CAD build for the part. Positions are in the model's coordinates, mm. A direction names the side the tool comes from. Give positions to 0.01 mm unless a question says otherwise; leave off trailing zeros. Order: outer loops, then holes, each group sorted by start corner. A loop starts at its lowest first (then second) coordinate and runs counter-clockwise, first axis right, second up. Notation, with made-up numbers: (-14, 30.5) -> (23, 30.5) arc R21 cw to (23, 44.5) -> close; hole circle Ø5 at (-5, 61.5). An arc over 180 degrees is marked (long way). Use one line per item in the form item = value. Start each with the question number.
1) Probe line 1 (X direction, y = 2.75, z = 50.8) (1 decimal); line 2 (Z direction, x = -35.5, y = 5.75). List the from-to ranges inside material, lowest first.
2) Mould opens along Z. For faces 3 (the face through (-41.275, 3, 5)), 4 (the face through (-0.7, 3.13, 24.87)), 5 (the face through (-34.213, 3.131, -40.322)), 6 (the face through (-23, 3, 55.562)) say: pulls with the +Z half, pulls with the -Z half, needs draft (parallel to the pull), parting line crosses it, or undercut.
3) Cut at A-A, the plane x = 0. Give the cut face in (y, z).
4) Cut at C-C, the plane y = 3.75. Give the cut face in (x, z) (1 decimal).
5) Tool access for faces 1 (the face through (0, 3, 46.038)), 2 (the face through (-35.364, 3.131, 53.008)): list every direction of +Z, -Z, +X, -X, +Y, -Y with a clear straight run to the whole face (end or side of a thin tool).
6) Cut at B-B, the plane z = 50.8. State how many separate pieces and enclosed holes the cut face has, and give its area (3 significant figures).
from build123d import *

# Parameters (mm, degrees)
SKETCH1_R           = 2.4892
SKETCH1_R_2         = 3.2512
BOSS_EXTRUDE1_DEPTH = 6.35


with BuildPart() as part:
    # Sketch1 → Boss-Extrude1 (new body)
    with BuildSketch(Plane(origin=(0, 0, 0), x_dir=(1, 0, 0), z_dir=(0, 1, 0))):
        Polygon((-41.275, 46.0375), (41.275, 46.0375), (41.275, -55.5625), (4.7625, -55.5625), (4.7625, -46.0375), (-4.7625, -46.0375), (-4.7625, -55.5625), (-41.275, -55.5625), align=None)
        with Locations((-36.5125, 41.275)):
            Circle(SKETCH1_R, mode=Mode.SUBTRACT)
        with Locations((36.5125, 41.275)):
            Circle(SKETCH1_R, mode=Mode.SUBTRACT)
        with Locations((36.5125, -50.8)):
            Circle(SKETCH1_R, mode=Mode.SUBTRACT)
        with Locations((-36.5125, -50.8)):
            Circle(SKETCH1_R, mode=Mode.SUBTRACT)
        with Locations((0, 12.170833333)):
            Circle(SKETCH1_R_2, mode=Mode.SUBTRACT)
        with Locations((0, -21.695833333)):
            Circle(SKETCH1_R_2, mode=Mode.SUBTRACT)
    extrude(amount=BOSS_EXTRUDE1_DEPTH)


solid = part.part
Result:
q1.line_1 = -41.3 to -39, -34 to -4.8, 4.8 to 34, 39 to 41.3
q1.line_2 = -46.04 to -43.55, -39 to 48.53, 53.07 to 55.56
q2.face_3 = needs draft
q2.face_4 = undercut
q2.face_5 = undercut
q2.face_6 = pulls with the +Z half
q3.outline = (0, -46.04) -> (6.35, -46.04) -> (6.35, -15.42) -> (0, -15.42) -> close; (0, -8.92) -> (6.35, -8.92) -> (6.35, 18.44) -> (0, 18.44) -> close; (0, 24.95) -> (6.35, 24.95) -> (6.35, 46.04) -> (0, 46.04) -> close
q4.outline = (-41.3, -46) -> (41.3, -46) -> (41.3, 55.6) -> (4.8, 55.6) -> (4.8, 46) -> (-4.8, 46) -> (-4.8, 55.6) -> (-41.3, 55.6) -> close; hole circle Ø5 at (-36.5, -41.3); hole circle Ø5 at (-36.5, 50.8); hole circle Ø6.5 at (0, -12.2); hole circle Ø6.5 at (0, 21.7); hole circle Ø5 at (36.5, -41.3); hole circle Ø5 at (36.5, 50.8)
q5.face_1 = +Z, +Y, -Y
q5.face_2 = +Y, -Y
q6.separate_pieces = 4
q6.enclosed_holes = 0
q6.area = 400 mm²
